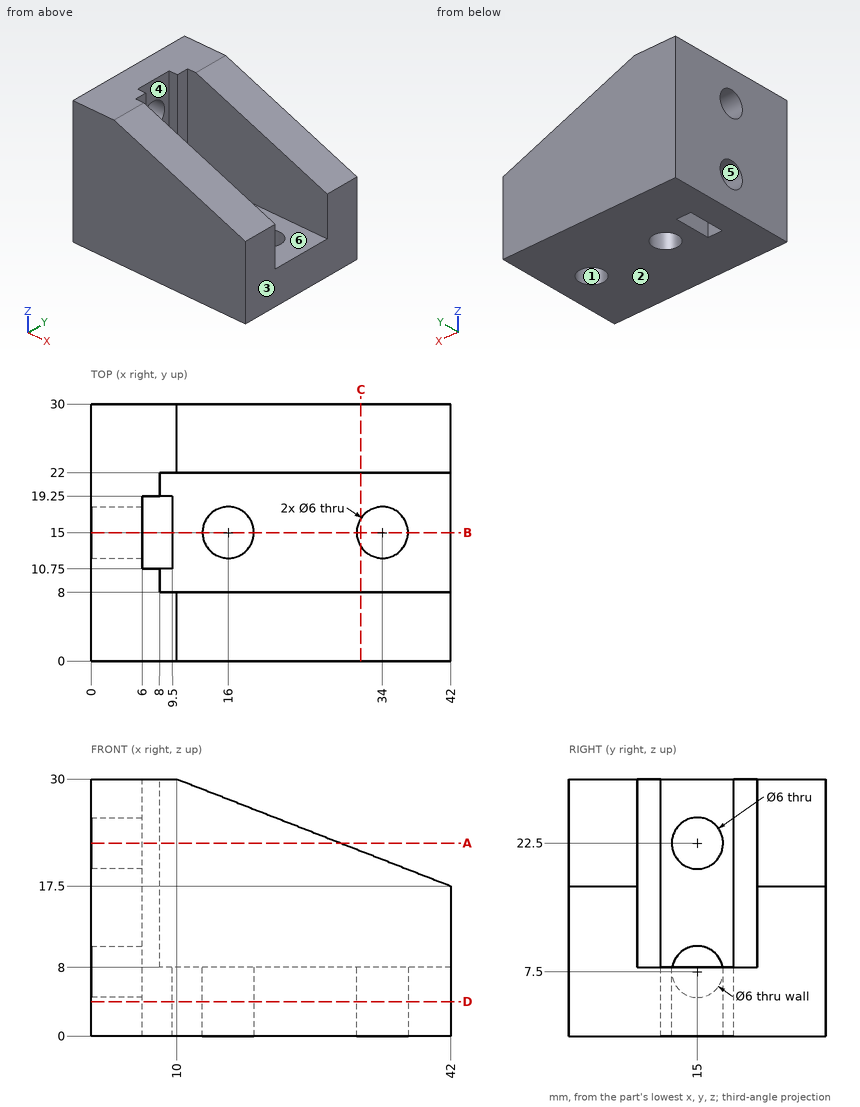
Could you check a few things on this drawing? It's one solid part, dimensions in mm from its lowest x, y, z. A direction names the side the tool comes from. Give positions to 0.01 mm unless a question says otherwise; leave off trailing zeros. Write each loop counter-clockwise with the first axis right and the second up, starting at its lowest first coordinate (ties: lowest second). Pieces come first, ordered by that corner, then holes. Notation, with made-up numbers: (9.5, 8) -> (62.5, 8) arc R29 ccw to (62.5, 40) -> close; hole circle Ø6 at (70, -16). An arc over 180 degrees is marked (long way). Answer as a JSON object with one key per item and string values.
Q1. Which directions (+Z, -Z, +X, -X, +Y, -Y) give clear straight access to the entire face, cutting with the end or side of a thin tool? Please do the marked faces 4, 5 and 6.
Taken from the geometry:
{"face 4": "+Z, -Z", "face 5": "-X", "face 6": "+Z, +X"}
Q2. Suppose I cut it at B-B on y = 15. Write out the boundary of the cut face in (x, z), then the cut area to 3 significant figures.
Taken from the geometry:
{"outline": "(0, 0) -> (6, 0) -> (6, 4.5) -> (0, 4.5) -> close; (0, 10.5) -> (6, 10.5) -> (6, 19.5) -> (0, 19.5) -> close; (0, 25.5) -> (6, 25.5) -> (6, 30) -> (0, 30) -> close; (9.5, 0) -> (13, 0) -> (13, 8) -> (9.5, 8) -> close; (19, 0) -> (31, 0) -> (31, 8) -> (19, 8) -> close; (37, 0) -> (42, 0) -> (42, 8) -> (37, 8) -> close", "area": "272 mm²"}
Q3. We'd pull the mould along X, two halves only. Please class the marked faces 1, 2 and 3: released by +X, released by -X, zero draft, split by the parting line, or undercut.
Taken from the geometry:
{"face 1": "undercut", "face 2": "zero draft", "face 3": "released by +X"}
Q4. Will these pins go through, and if not, where does the flat tip stop? pin 1 Ø3.5 at (y, z) = (15, 22.5) entering from +X; pin 2 Ø7 at (y, z) = (13, 14.5) entering from +X; pin 3 Ø6 at (y, z) = (11, 9) entering from +X; pin 4 Ø4 at (x, y) = (30.5, 13.5) entering from +Z.
Taken from the geometry:
{"pin 1": "passes through", "pin 2": "stops at x = 8", "pin 3": "stops at x = 42", "pin 4": "stops at z = 8"}
Q5. Suppose I cut it at A-A on z = 22.5. Write out the boundary of the cut face in (x, y).
Taken from the geometry:
{"outline": "(0, 0) -> (29.2, 0) -> (29.2, 8) -> (8, 8) -> (8, 10.75) -> (6, 10.75) -> (6, 12) -> (0, 12) -> close; (0, 18) -> (6, 18) -> (6, 19.25) -> (8, 19.25) -> (8, 22) -> (29.2, 22) -> (29.2, 30) -> (0, 30) -> close"}
Q6. Suppose I cut it at C-C on x = 31.5. Write out the boundary of the cut face in (y, z), then the cut area to 3 significant figures.
Taken from the geometry:
{"outline": "(0, 0) -> (13.34, 0) -> (13.34, 8) -> (8, 8) -> (8, 21.6) -> (0, 21.6) -> close; (16.66, 0) -> (30, 0) -> (30, 21.6) -> (22, 21.6) -> (22, 8) -> (16.66, 8) -> close", "area": "431 mm²"}
Q7. Suppose I cut it at D-D on z = 4. Write out the boundary of the cut face in (x, y), then the cut area to 3 significant figures.
Taken from the geometry:
{"outline": "(0, 0) -> (42, 0) -> (42, 30) -> (0, 30) -> close; hole (6, 10.75) -> (9.5, 10.75) -> (9.5, 19.25) -> (6, 19.25) -> close; hole circle Ø6 at (16, 15); hole circle Ø6 at (34, 15)", "area": "1,170 mm²"}
Q8. Please list where these lines run through material, in increasing order: L1, parallel to Y at x = 16, z = 24.5; L2, parallel to Y at x = 3, z = 22.5; L3, parallel to Z at x = 31, y = 21.
Taken from the geometry:
{"L1": "y = 0 to 8, 22 to 30", "L2": "y = 0 to 12, 18 to 30", "L3": "z = 0 to 8"}
